Read the model definition and answer for the solid it produces. Units are mm, in the model's axes. A direction names the side the tool comes from. Give positions to 0.01 mm unless a question says otherwise; leave off trailing zeros. Write each loop counter-clockwise with the first axis right and the second up, starting at its lowest first coordinate (ties: lowest second). Pieces come first, ordered by that corner, then holes. Notation, with made-up numbers: M 72.5,5 L 91.5,5 A21 cw 91.5,18 Z; hole C -20.5,68.5 d7. An arc over 180 degrees is marked long. Write each question's results on one line, items separated by ' | '. Start each with the question number.
```python
from build123d import *

# Parameters (mm, degrees)
SKETCH1_R           = 5
BOSS_EXTRUDE1_DEPTH = 5
SKETCH2_W           = 59.402785504
SKETCH2_H           = 20
CUT_EXTRUDE1_DEPTH  = 136.462171841


with BuildPart() as part:
    # Sketch1 → Boss-Extrude1 (new, symmetric)
    with BuildSketch(Plane.XY):
        with BuildLine():
            Line((0, 10), (125, 10))
            ThreePointArc((125, 10), (135, 0), (125, -10))
            Line((125, -10), (0, -10))
            ThreePointArc((0, -10), (-10, 0), (0, 10))
        make_face()
        Circle(SKETCH1_R, mode=Mode.SUBTRACT)
        with Locations((125, 0)):
            Circle(SKETCH1_R, mode=Mode.SUBTRACT)
    extrude(amount=BOSS_EXTRUDE1_DEPTH, both=True)

    # Sketch2 → Cut-Extrude1 (cut, through all)
    with BuildSketch(Plane.XY):
        with Locations((0.298607248, 0)):
            Rectangle(SKETCH2_W, SKETCH2_H)
    extrude(amount=-CUT_EXTRUDE1_DEPTH, mode=Mode.SUBTRACT)


solid = part.part
```
Item 1: Determine the mould class of faces 3 (the cylindrical face through (-10, 0, 3)), 4 (the flat face through (62, 10, 0)), 5 (the cylindrical face through (129.77, 1.5, -0.07)) for opening direction Y: +Y half, -Y half, draft (parallel to the pull), parting line (faces both ways), or undercut.
Item 2: Given P1, Ø2, axis at y = -3.5, z = 2.5, coming from the -X side; P2, Ø1, axis at y = 6.5, z = -3.5, coming from the -X side; P3, Ø6, axis at x = 0, y = 0, coming from the -Z side; P4, Ø1, axis at y = -8, z = 1.5, coming from the -X side, each flat-ended and moving along its own axis, determine where each tip first touches the part or whether it passes through.
Item 3: Section D-D, the plane x = 15.5 is taken. Determine the outline of the cut face in (y, z).
Item 4: Section B-B, the plane z = 3.75 is taken. Determine the outline of the cut face in (x, y).
Item 5: For faces 1 (the flat face through (14, 0, 0)), 2 (the cylindrical face through (135, 0, 0)), determine the directions among +Z, -Z, +X, -X, +Y, -Y from which every point of the face is accessible in a straight line to the end or side of a thin tool.
Item 6: Section C-C, the plane z = -2 is taken. Determine the outline of the cut face in (x, y).
Item 7: Straight lines are drawn through the part: line 1 (X direction, y = 0.25, z = 3.75); line 2 (Y direction, x = 0, z = 2.05); line 3 (X direction, y = -2.5, z = 1). For each, find the intervals that lie inside material, in ascending order.
Item 8: Section A-A, the plane y = 0 is taken. Determine the outline of the cut face in (x, z), then the cut area to 3 significant figures.
Worked out:
1) face 3: parting line | face 4: +Y half | face 5: undercut
2) P1: stops at x = -9.68 | P2: stops at x = 30 | P3: passes through | P4: stops at x = -6.61
3) outline: M -10,0 L 10,0 L 10,5 L -10,5 Z
4) outline: M 0,-10 L 125,-10 A10 ccw 125,10 L 0,10 A10 ccw Z; hole C 0,0 d10; hole C 125,0 d10
5) face 1: -Z, -X, +Y, -Y | face 2: +Z, -Z, +X
6) outline: M 30,-10 L 125,-10 A10 ccw 125,10 L 30,10 Z; hole C 125,0 d10
7) line 1: x = -10 to -4.99, 4.99 to 120.01, 129.99 to 135 | line 2: y = -10 to -5, 5 to 10 | line 3: x = -9.68 to -4.33, 4.33 to 120.67, 129.33 to 134.68
8) outline: M -10,0 L -5,0 L -5,5 L -10,5 Z; M 5,0 L 30,0 L 30,-5 L 120,-5 L 120,5 L 5,5 Z; M 130,-5 L 135,-5 L 135,5 L 130,5 Z | area: 1,100 mm²
